Here's how the part is built. I have some questions about the finished solid (model axes, mm). A direction names the side the tool comes from. Round coordinates to 2 decimals unless told otherwise and drop trailing zeros. Order: outer loops, then holes, each group sorted by start corner. A loop starts at its lowest first (then second) coordinate and runs counter-clockwise, first axis right, second up. Notation, with made-up numbers: M -11.75,71 L 23.25,71 A15 ccw 23.25,95 Z; hole C 17.5,20.25 d10. An arc over 180 degrees is marked long. Write item = value, one per line. Start each with the question number.
Item 1: I want a section at B-B, the plane x = 0. List the corners of the cut face in (y, z) for me.
Item 2: I want a section at C-C, the plane z = 0. List the corners of the cut face in (x, y) for me.
Item 3: We'd pull the mould along Z, two halves only. Please class faces 1 (the face through (-9.76, 2.96, -2.17)), 2 (the face through (11.413, 2.104, -11.214)), 3 (the face through (0.2, 0, 10.3)): pulls with the +Z half, pulls with the -Z half, needs draft (parallel to the pull), parting line crosses it, or undercut.
Item 4: Please list where these lines run through material, in increasing order: L1, parallel to X at y = 4.6, z = 0; L2, parallel to Z at x = -3.5, y = 5.45; L3, parallel to Z at x = -3, y = 2.2.
Item 5: I want a section at A-A, the plane y = 0.8. List the corners of the cut face in (x, z) for me.
Item 6: For faces 4 (the face through (-15, 3, 2.5)), 5 (the face through (-2.5, 3, 15)), 6 (the face through (-2.5, 3, -15)), 7 (the face through (15, 3, -2.5)), which set-ups out of +Z, -Z, +X, -X, +Y, -Y let a thin tool reach every point of the face, with its end or its side?
Item 7: I'm going to push flat-ended pins straight in: P1, Ø3, axis at y = 3.5, z = 5, coming from the -X side; P2, Ø2.5, axis at y = 4, z = 1, coming from the -X side; P3, Ø0.5, axis at x = -15, y = 2, coming from the +Z side. Where does each tip first touch, or does it pass through?
```python
from build123d import *

# Parameters (mm, degrees)
CROQUIS1_R              = 16
CROQUIS1_R_2            = 10
SALIENTE_EXTRUIR1_DEPTH = 6
CROQUIS2_W              = 5
CROQUIS2_H              = 2
CROQUIS2_W_2            = 2
CROQUIS2_H_2            = 5
CORTAR_EXTRUIR1_DEPTH   = 6


with BuildPart() as part:
    # Croquis1 → Saliente-Extruir1 (new body)
    with BuildSketch(Plane(origin=(0, 0, 0), x_dir=(1, 0, 0), z_dir=(0, 1, 0))):
        with Locations(Location((0, 0, 0), (0, 0, 270))):
            Circle(CROQUIS1_R)
        with Locations(Location((0, 0, 0), (0, 0, 270))):
            Circle(CROQUIS1_R_2, mode=Mode.SUBTRACT)
    extrude(amount=SALIENTE_EXTRUIR1_DEPTH)

    # Croquis2 → Cortar-Extruir1 (cut)
    with BuildSketch(Plane(origin=(0, 6, 0), x_dir=(1, 0, 0), z_dir=(0, 1, 0))):
        with Locations((0, 15)):
            Rectangle(CROQUIS2_W, CROQUIS2_H)
        with Locations((0, -15)):
            Rectangle(CROQUIS2_W, CROQUIS2_H)
        with Locations((15, 0)):
            Rectangle(CROQUIS2_W_2, CROQUIS2_H_2)
        with Locations((-15, 0)):
            Rectangle(CROQUIS2_W_2, CROQUIS2_H_2)
    extrude(amount=-CORTAR_EXTRUIR1_DEPTH, mode=Mode.SUBTRACT)

    # Croquis3 → Cortar-Revolución1 (revolve, cut)
    with BuildSketch(Plane(origin=(0, 0, 0), x_dir=(0, 0, -1), z_dir=(1, 0, 0)), mode=Mode.PRIVATE) as cortar_revoluci_n1_sk:
        Polygon((-16, 6), (-13, 6), (-16, 4.267949192), align=None)
    revolve(cortar_revoluci_n1_sk.sketch.rotate(Axis((0, 6, 0), (0, -1, 0)), 171.010700805), axis=Axis((0, 6, 0), (0, -1, 0)), mode=Mode.SUBTRACT)


solid = part.part
```
Filled in:
q1.outline = M 0,-14 L 5.42,-14 L 6,-13 L 6,-10 L 0,-10 Z; M 0,10 L 6,10 L 6,13 L 5.42,14 L 0,14 Z
q2.outline = M -14,0 L -10,0 L -10,6 L -13,6 L -14,5.42 Z; M 10,0 L 14,0 L 14,5.42 L 13,6 L 10,6 Z
q3.face_1 = undercut
q3.face_2 = pulls with the -Z half
q3.face_3 = needs draft
q4.L1 = -14 to -10, 10 to 14
q4.L2 = -13.51 to -9.37, 9.37 to 13.51
q4.L3 = -15.72 to -9.54, 9.54 to 15.72
q5.outline = M -15.8,-2.5 A16 ccw -2.5,-15.8 L -2.5,-14 L 2.5,-14 L 2.5,-15.8 A16 ccw 15.8,-2.5 L 14,-2.5 L 14,2.5 L 15.8,2.5 A16 ccw 2.5,15.8 L 2.5,14 L -2.5,14 L -2.5,15.8 A16 ccw -15.8,2.5 L -14,2.5 L -14,-2.5 Z; hole C 0,0 d20
q6.face_4 = -X, +Y, -Y
q6.face_5 = +Z, +Y, -Y
q6.face_6 = -Z, +Y, -Y
q6.face_7 = +X, +Y, -Y
q7.P1 = -15.61
q7.P2 = -14
q7.P3 = 6.2
